```python
from build123d import *

# Parameters (mm, degrees)
F0_W     = 100
F0_H     = 100
F0_R     = 40
F0_R_2   = 35
F1_DEPTH = 5
F2_DEPTH = 50
F3_R     = 7.5
F4_DEPTH = 80
F6_DEPTH = 25


with BuildPart() as f1:
    # F0 (on Top) → F1 (new body)
    with BuildSketch(Plane.XY):
        Rectangle(F0_W, F0_H)
        Circle(F0_R, mode=Mode.SUBTRACT)
        Circle(F0_R)
        Circle(F0_R_2, mode=Mode.SUBTRACT)
        Circle(F0_R_2)
    extrude(amount=-F1_DEPTH)

    # F0 (on Top) → F2 (join)
    with BuildSketch(Plane.XY):
        Circle(F0_R)
        Circle(F0_R_2, mode=Mode.SUBTRACT)
    extrude(amount=F2_DEPTH)

    # F3 (on face) → F4 (join)
    with BuildSketch(Plane(origin=(0, 0, -5), x_dir=(1, 0, 0), z_dir=(0, 0, -1))):
        Circle(F3_R)
    extrude(amount=F4_DEPTH)


with BuildPart() as f6:
    # F5 (on Front) → F6 (new body, symmetric)
    with BuildSketch(Plane.XZ):
        Polygon((13.101274, -90.236664), (13.101274, -61.807115), (-15.328275, -90.236664), align=None)
    extrude(amount=F6_DEPTH, both=True)


with BuildPart() as f1_1:
    add(f1.part)

    # F7: cut F6
    add(f6.part, mode=Mode.SUBTRACT)


solid = f1_1.part
```
The listing builds one solid part. Answer for the finished solid, in the listing's coordinates (mm). A direction names the side the tool comes from. Round coordinates to 2 decimals unless told otherwise and drop trailing zeros. Loops run counter-clockwise (first coordinate to the right, second up) from the corner with the lowest first, then second, coordinate; pieces in that order, holes last.
Q1. Section A-A, the plane z = 8 is taken. Determine the outline of the cut face in (x, y).
Q2. Find the intervals of material crossed by line 1 (Y direction, x = 0, z = 30); line 2 (Z direction, x = 7.5, y = -17); line 3 (Z direction, x = -31, y = -24), in increasing order.
Q3. Section C-C, the plane x = 38 is taken. Determine the outline of the cut face in (y, z), then the cut area to 3 significant figures.
Q4. Section B-B, the plane y = 13 is taken. Determine the outline of the cut face in (x, z), then the cut area to 3 significant figures.
Q5. Given pin 1 Ø8 at (y, z) = (7.5, -17.5) entering from -X; pin 2 Ø6 at (x, z) = (4, -65.5) entering from +Y; pin 3 Ø1.5 at (x, y) = (7.5, 5.5) entering from -Z; pin 4 Ø6 at (x, y) = (-28.5, 19.5) entering from +Z, each flat-ended and moving along its own axis, determine where each tip first touches the part or whether it passes through.
Q6. For a pull along Y with two mould halves and no side action, classify faces 1 (the face through (0, 0, 0)), 2 (the face through (-7.493, -0.33, -43.316)), 3 (the face through (-1, 50, -2)), 4 (the face through (-28, -21, 25)) as released by +Y, released by -Y, zero draft, split by the parting line, or undercut.
Q7. Section D-D, the plane z = -31.5 is taken. Determine the outline of the cut face in (x, y).
Q8. Which of the six approach directions +Z, -Z, +X, -X, +Y, -Y give full straight-line access (tool end or side, diameter ignored) to faces 5 (the face through (-1, -50, -2)), 6 (the face through (-34, 23, 0))?
Completed:
1. outline: circle Ø80 at (0, 0); hole circle Ø70 at (0, 0)
2. line 1: y = -40 to -35, 35 to 40
2. line 2: z = -5 to 0
2. line 3: z = -5 to 50
3. outline: (-50, -5) - (50, -5) - (50, 0) - (12.49, 0) - (12.49, 50) - (-12.49, 50) - (-12.49, 0) - (-50, 0) - close
3. area: 1,750 mm2
4. outline: (-50, -5) - (50, -5) - (50, 0) - (37.83, 0) - (37.83, 50) - (32.5, 50) - (32.5, 0) - (-32.5, 0) - (-32.5, 50) - (-37.83, 50) - (-37.83, 0) - (-50, 0) - close
4. area: 1,030 mm2
5. pin 1: stops at x = -6.63
5. pin 2: stops at y = 7.43
5. pin 3: stops at z = -5
5. pin 4: stops at z = 50
6. face 1: undercut
6. face 2: split by the parting line
6. face 3: released by +Y
6. face 4: undercut
7. outline: circle Ø15 at (0, 0)
8. face 5: +Z, -Z, +X, -X, -Y
8. face 6: +Z
